Work out the finished part from the listing and answer in its coordinate system (mm). A direction names the side the tool comes from. Round coordinates to 2 decimals unless told otherwise and drop trailing zeros. Order: outer loops, then holes, each group sorted by start corner. A loop starts at its lowest first (then second) coordinate and runs counter-clockwise, first axis right, second up. Notation, with made-up numbers: M 68,16 L 109,16 A20 cw 109,44 Z; hole C 14,23.5 d5. An arc over 180 degrees is marked long. Return JSON: item names as keys, results as strings.
from build123d import *

# Parameters (mm, degrees)
BOSS_EXTRUDE1_DEPTH = 2
FILLET1_R           = 1
FILLET2_R           = 5
FILLET3_R           = 9
BOSS_EXTRUDE2_DEPTH = 2
SKETCH3_W           = 1.5
SKETCH3_H           = 25
CUT_EXTRUDE1_DEPTH  = 2


with BuildPart() as part:
    # Sketch1 → Boss-Extrude1 (new body)
    with BuildSketch(Plane(origin=(0, 0, 0), x_dir=(1, 0, 0), z_dir=(0, 1, 0))):
        Polygon((3, 0), (5, 0), (10, 11.071428571), (15, 0), (17, 0), (17, -5), (20, -5), (20, 0), (20, 2), (13, 17.5), (20, 33), (20, 35), (20, 40), (17, 40), (17, 35), (15, 35), (10, 23.928571429), (5, 35), (3, 35), (3, 40), (0, 40), (0, 35), (0, 33), (7, 17.5), (0, 2), (0, 0), (0, -5), (3, -5), align=None)
    extrude(amount=BOSS_EXTRUDE1_DEPTH)

    # Fillet1
    fillet1_edges = [part.edges().sort_by_distance(p)[0] for p in [
        (10, 1, -23.928571429),
        (10, 1, -11.071428571),
    ]]
    fillet(fillet1_edges, radius=FILLET1_R)

    # Fillet2
    fillet2_edges = [part.edges().sort_by_distance(p)[0] for p in [
        (7, 1, -17.5),
        (13, 1, -17.5),
    ]]
    fillet(fillet2_edges, radius=FILLET2_R)

    # Fillet3
    fillet3_edges = [part.edges().sort_by_distance(p)[0] for p in [
        (0, 1, -2),
        (0, 1, -33),
        (20, 1, -33),
        (20, 1, -2),
    ]]
    fillet(fillet3_edges, radius=FILLET3_R)

    # Sketch2 → Boss-Extrude2 (add)
    with BuildSketch(Plane(origin=(0, 2, 0), x_dir=(1, 0, 0), z_dir=(0, 1, 0))):
        Polygon((3, 35), (0, 35), (0, 0), (3, 0), (9.069161159, 17.5), align=None)
    extrude(amount=-BOSS_EXTRUDE2_DEPTH)

    # Sketch3 → Cut-Extrude1 (cut)
    with BuildSketch(Plane(origin=(0, 2, 0), x_dir=(1, 0, 0), z_dir=(0, 1, 0))):
        with Locations((3.25, 17.5)):
            Rectangle(SKETCH3_W, SKETCH3_H)
    extrude(amount=-CUT_EXTRUDE1_DEPTH, mode=Mode.SUBTRACT)


solid = part.part
Item 1: Consider line 1 along Z through (x, y) = (2.75, 1.8); line 2 along X through (y, z) = (1.3, -8); line 3 along X through (y, z) = (1.2, -9). Determine where each line is inside the solid, lowest interval first. Write a range as [from, to].
Output:
{"line 1": "z = [-40, -30], [-5, 5]", "line 2": "x = [0, 2.5], [4, 8.61], [11.39, 17.29]", "line 3": "x = [0, 2.5], [4, 9.06], [10.94, 16.84]"}
Item 2: Which of the six approach directions +Z, -Z, +X, -X, +Y, -Y give full straight-line access (tool end or side, diameter ignored) to faces 1 (the flat face through (2.5, 1, -17)), 2 (the flat face through (7.016, 0.986, -4.463)), 3 (the flat face through (16, 1, -35)), 4 (the flat face through (16.603, 0.986, -9.522)), 5 (the flat face through (20, 1, 3))?
Output:
{"face 1": "+Y, -Y", "face 2": "+Z, +Y, -Y", "face 3": "-Z, +Y, -Y", "face 4": "+X, +Y, -Y", "face 5": "+Z, -Z, +X, +Y, -Y"}
Item 3: The mould has two halves that part along X. Classify faces 6 (the flat face through (17, 1, 2)), 7 (the cylindrical face through (19.804, 1.014, -1.93)), 8 (the flat face through (19, 1, -40)): pulls with the +X half, pulls with the -X half, needs draft (parallel to the pull), parting line crosses it, or undercut.
Output:
{"face 6": "undercut", "face 7": "pulls with the +X half", "face 8": "needs draft"}
Item 4: Find section D-D (z = -26.5). Determine the outline of the cut face in (x, y).
Output:
{"outline": "M 0,0 L 2.5,0 L 2.5,2 L 0,2 Z; M 4,0 L 8.84,0 L 8.84,2 L 4,2 Z; M 11.16,0 L 17.06,0 L 17.06,2 L 11.16,2 Z"}
Item 5: Find section B-B (x = 16.5). Determine the outline of the cut face in (y, z).
Output:
{"outline": "M 0,-35 L 2,-35 L 2,-25.25 L 0,-25.25 Z; M 0,-9.75 L 2,-9.75 L 2,0 L 0,0 Z"}
Item 6: Find section C-C (z = -36). Determine the outline of the cut face in (x, y), plus the area to 3 significant figures.
Output:
{"outline": "M 0,0 L 3,0 L 3,2 L 0,2 Z; M 17,0 L 20,0 L 20,2 L 17,2 Z", "area": "12.0 mm^2"}
Item 7: Each of these flat-tipped pins is pushed along its axis until it touches: pin 1 (0.8 mm diameter, centred on x = 3.5, y = 1, fed in from -Z); pin 2 (1 mm diameter, centred on x = 15.5, y = 0.5, fed in from +Z). Where does it stop, or does it pass through?
Output:
{"pin 1": "stops at z = -35", "pin 2": "stops at z = 0"}
